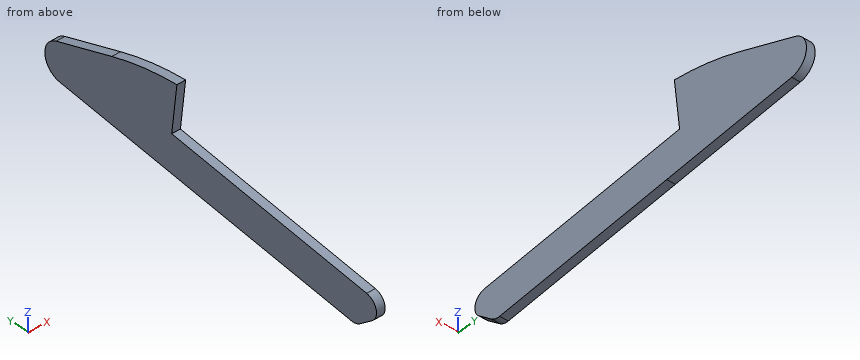
```python
from build123d import *

# Parameters (mm, degrees)
F1_DEPTH = 4.445


with BuildPart() as f1:
    # F0 (on Right) → F1 (new body)
    with BuildSketch(Plane.YZ):
        with BuildLine():
            Line((-71.929009, 10.879191), (-103.618976, 21.664825))
            ThreePointArc((-103.618976, 21.664825), (-121.890076, 26.640612), (-140.637203, 29.312091))
            Line((-140.637203, 29.312091), (-137.672003, 4.085764))
            Line((-137.672003, 4.085764), (-248.578204, -8.950579))
            ThreePointArc((-248.578204, -8.950579), (-253.947109, -13.528608), (-251.772153, -20.240766))
            Line((-251.772153, -20.240766), (-244.724271, -25.806048))
            ThreePointArc((-244.724271, -25.806048), (-242.517575, -26.932648), (-240.047723, -27.129024))
            Line((-240.047723, -27.129024), (-145.021622, -15.95929))
            Line((-145.021622, -15.95929), (-73.886, -7.597734))
            ThreePointArc((-73.886, -7.597734), (-65.525931, 0.858906), (-71.929009, 10.879191))
        make_face()
    extrude(amount=F1_DEPTH)


solid = f1.part
```
Design review of the part built by this model. Coordinates are the model's own, in mm. Round coordinates to 2 decimals unless told otherwise and drop trailing zeros. Write each loop counter-clockwise with the first axis right and the second up, starting at its lowest first coordinate (ties: lowest second). Pieces come first, ordered by that corner, then holes. Notation, with made-up numbers: (41.25, 71) -> (52.25, 71) arc R26 ccw to (52.25, 98) -> close; hole circle Ø7 at (2.25, -3). An arc over 180 degrees is marked (long way). Write item = value, one per line. Start each with the question number.
1) Wall thickness on probe 1 along Y at (x, z) = (2.65, 8); probe 2 along Z at (x, y) = (1.25, -204); probe 3 along Y at (x, z) = (0.65, 10): over which ranges is each line inside the solid? List them lowest first. Write a range as from..to.
2) Take a section at A-A, the plane x = 1.85. State the section outline as (y, z) points (3 decimals).
3) Clearance check with flat-ended pins moving along their axes: pin 1 (1 mm diameter, centred on x = 4, y = -203, fed in from +Z); pin 2 (2 mm diameter, centred on x = 3, y = -139, fed in from -Z); pin 3 (1.5 mm diameter, centred on x = 4, y = -88, fed in from +Z). State where each tip first meets the part, or that it passes through.
4) Take a section at C-C, the plane y = -120.5. State the section outline as (x, z) points (3 decimals).
5) Take a section at B-B, the plane z = -24. State the section outline as (x, y) points (3 decimals).
Results list:
q1.probe_1 = -138.13..-67.71
q1.probe_2 = -22.89..-3.71
q1.probe_3 = -138.37..-70.05
q2.outline = (-251.772, -20.241) -> (-244.724, -25.806) arc R6.35 ccw to (-240.048, -27.129) -> (-73.886, -7.598) arc R9.525 ccw to (-71.929, 10.879) -> (-103.619, 21.665) arc R152.4 ccw to (-140.637, 29.312) -> (-137.672, 4.086) -> (-248.578, -8.951) arc R6.35 ccw to start
q3.pin_1 = -3.53
q3.pin_2 = -15.37
q3.pin_3 = 16.6
q4.outline = (0, -13.077) -> (4.445, -13.077) -> (4.445, 26.347) -> (0, 26.347) -> close
q5.outline = (0, -247.011) -> (4.445, -247.011) -> (4.445, -213.428) -> (0, -213.428) -> close
